from build123d import *

# Parameters (mm, degrees)
EXTRUDE_1_DEPTH     = 15
REVOLVE_1_ANGLE     = 180.0000000000004
CUT_EXTRUDE_START   = -19
CUT_EXTRUDE_1_DEPTH = 19
SKETCH_5_R          = 10
CUT_EXTRUDE_2_DEPTH = 87.34958022017247
SKETCH_4_R          = 1.2499999999999991
SKETCH_4_R_2        = 1.2500000000000002
SKETCH_4_R_3        = 1.2499999999999996
SKETCH_4_R_4        = 1.2499999999999987
SKETCH_4_R_5        = 1.2499999999999984
SKETCH_4_R_6        = 1.249999999999999
SKETCH_4_R_7        = 5.1000000000000005
CUT_EXTRUDE_3_DEPTH = 86.88509768172823
CUT_EXTRUDE_START_2 = -3
CUT_EXTRUDE_5_DEPTH = 3
SKETCH_6_R          = 6.200000000000004
CUT_EXTRUDE_4_DEPTH = 4.2
EXTRUDE_2_DEPTH     = 15
CHAMFER_1_SIZE      = 0.3
HOLE_WIZARD_1_D     = 1.7
HOLE_WIZARD_1_DEPTH = 3.5


with BuildPart() as part:
    # 草图2 → 凸台-拉伸1 (new body)
    with BuildSketch(Plane(origin=(0, 0, 0), x_dir=(1, 0, 0), z_dir=(0, 1, 0))):
        with BuildLine():
            Line((70.44642857142858, 12.492025517529665), (0.5357142857142793, 14.990430621035568))
            ThreePointArc((0.5357142857142791, 14.990430621035566), (-10.41547612244118, 10.79434375693384), (-14.99999999999997, 1.22e-15))
            Line((-15, 0), (82.5, -8.67e-15))
            ThreePointArc((82.5, -8.44e-15), (78.99528646411157, 8.679563435367664), (70.44642857142858, 12.492025517529667))
        make_face()
        with BuildLine():
            Line((82.5, -8.67e-15), (-15, 0))
            ThreePointArc((-14.999999999999998, 0), (-10.415476122441204, -10.794343756933866), (0.535714285714286, -14.990430621035598))
            Line((0.5357142857142848, -14.990430621035598), (70.44642857142858, -12.492025517529669))
            ThreePointArc((70.44642857142858, -12.492025517529669), (78.99528646411156, -8.679563435367672), (82.5, -8.72e-15))
        make_face()
    extrude(amount=EXTRUDE_1_DEPTH)

    # 草图1 → 旋转1 (revolve)
    with BuildSketch(Plane(origin=(0, 0, 0), x_dir=(1, 0, 0), z_dir=(0, 1, 0))):
        with BuildLine():
            Line((0.5357142857142848, -14.990430621035598), (70.44642857142858, -12.492025517529669))
            ThreePointArc((70.44642857142858, -12.492025517529669), (78.99528646411156, -8.67956343536767), (82.5, 0))
            Line((82.5, 0), (-15, 0))
            ThreePointArc((-15, 0), (-10.415476122441207, -10.794343756933864), (0.5357142857142848, -14.990430621035598))
        make_face()
    revolve(axis=Axis((70, 0, 8.67e-15), (1, 0, 1.2e-16)), revolution_arc=REVOLVE_1_ANGLE)

    # 草图3 → 切除-拉伸1 (cut)
    with BuildSketch(Plane(origin=(0, 15, 0), x_dir=(1, 0, 0), z_dir=(0, 1, 0)).offset(CUT_EXTRUDE_START)):
        with BuildLine():
            Line((17.295525226029294, 14.391483841348133), (0.5357142857142793, 14.990430621035568))
            ThreePointArc((0.5357142857142793, 14.990430621035568), (-14.999999999999972, 1.84e-15), (0.5357142857142814, -14.990430621035584))
            Line((0.5357142857142814, -14.990430621035584), (17.29552522602928, -14.391483841348148))
            ThreePointArc((17.29552522602928, -14.391483841348148), (22.5, -9.99e-15), (17.295525226029294, 14.391483841348133))
        make_face()
    extrude(amount=CUT_EXTRUDE_1_DEPTH, mode=Mode.SUBTRACT)

    # 草图5 → 切除-拉伸2 (cut, through all)
    with BuildSketch(Plane(origin=(0, -6, 0), x_dir=(1, 0, 0), z_dir=(0, 1, 0))):
        with Locations(Location((0, 0, 0), (0, 0, 270))):
            Circle(SKETCH_5_R)
    extrude(amount=-CUT_EXTRUDE_2_DEPTH, mode=Mode.SUBTRACT)

    # 草图4 → 切除-拉伸3 (cut, through all)
    with BuildSketch(Plane(origin=(0, -4, 0), x_dir=(1, 0, 0), z_dir=(0, 1, 0))):
        with Locations(Location((8, 0, 0), (0, 0, 270))):
            Circle(SKETCH_4_R)
        with Locations(Location((5.656854249492371, -5.656854249492391, 0), (0, 0, 270))):
            Circle(SKETCH_4_R_2)
        with Locations(Location((-2.793e-14, -8, 0), (0, 0, 270))):
            Circle(SKETCH_4_R_3)
        with Locations(Location((-5.656854249492411, -5.65685424949235, 0), (0, 0, 270))):
            Circle(SKETCH_4_R_4)
        with Locations(Location((-8, 5.586e-14, 0), (0, 0, 270))):
            Circle(SKETCH_4_R_5)
        with Locations(Location((-5.65685424949233, 5.656854249492429, 0), (0, 0, 270))):
            Circle(SKETCH_4_R_3)
        with Locations(Location((8.38e-14, 7.999999999999998, 0), (0, 0, 270))):
            Circle(SKETCH_4_R_6)
        with Locations(Location((5.656854249492451, 5.656854249492311, 0), (0, 0, 270))):
            Circle(SKETCH_4_R_6)
        with Locations(Location((0, 0, 0), (0, 0, 270))):
            Circle(SKETCH_4_R_7)
    extrude(amount=-CUT_EXTRUDE_3_DEPTH, mode=Mode.SUBTRACT)

    # 草图11 → 切除-拉伸5 (cut)
    with BuildSketch(Plane(origin=(0, 15, 0), x_dir=(1, 0, 0), z_dir=(0, 1, 0)).offset(CUT_EXTRUDE_START_2)):
        with BuildLine():
            Line((60.46530800021301, 12.848721666733917), (70.44642857142858, 12.492025517529665))
            ThreePointArc((70.44642857142858, 12.492025517529665), (82.5, -8.67e-15), (70.44642857142858, -12.492025517529669))
            Line((70.44642857142858, -12.492025517529669), (60.46530800021299, -12.848721666733926))
            ThreePointArc((60.46530800021299, -12.848721666733926), (54, 3.9e-16), (60.46530800021301, 12.848721666733917))
        make_face()
    extrude(amount=CUT_EXTRUDE_5_DEPTH, mode=Mode.SUBTRACT)

    # 草图6 → 切除-拉伸4 (cut)
    with BuildSketch(Plane(origin=(0, 12, 0), x_dir=(1, 0, 0), z_dir=(0, 1, 0))):
        with Locations(Location((70, -8.67e-15, 0), (0, 0, 270))):
            Circle(SKETCH_6_R)
    extrude(amount=-CUT_EXTRUDE_4_DEPTH, mode=Mode.SUBTRACT)

    # 草图12 → 凸台-拉伸2 (add)
    with BuildSketch(Plane(origin=(0, 15, 0), x_dir=(1, 0, 0), z_dir=(0, 1, 0))):
        Polygon((38.755416613121156, 10.122335609132724), (38.59470232740688, 5.625206422822045), (46.58959865862586, 5.339492137107765), (46.750312944340145, 9.836621323418441), align=None)
        Polygon((30.760520281902174, 10.408049894847004), (30.59980599618789, 5.910920708536326), (38.59470232740688, 5.625206422822045), (38.755416613121156, 10.122335609132724), align=None)
    extrude(amount=EXTRUDE_2_DEPTH)

    # 倒角1
    chamfer_1_edges = [part.edges().sort_by_distance(p)[0] for p in [
        (38.755416613121156, 30, -10.122335609132723),
        (30.680163139045032, 30, -8.159485301691664),
        (38.59470232740688, 30, -5.625206422822045),
        (46.669955801483, 30, -7.588056730263103),
    ]]
    chamfer(chamfer_1_edges, length=CHAMFER_1_SIZE)

    # 孔1
    with Locations(Plane(origin=(0.41071428571427876, 0, -11.492663476127266), x_dir=(-0.9993620414023731, 0, -0.03571428571428518), z_dir=(0.03571428571428518, 0, -0.9993620414023731))):
        with Locations((-41.369180272, 27.499999998), (-35.369180272, 27.499999998)):
            Hole(HOLE_WIZARD_1_D / 2, depth=HOLE_WIZARD_1_DEPTH)


solid = part.part
Geometry check sheet. Reference: the model listing, model coordinates, mm. A direction names the side the tool comes from. Give positions to 0.01 mm unless a question says otherwise; leave off trailing zeros. Write each loop counter-clockwise with the first axis right and the second up, starting at its lowest first coordinate (ties: lowest second). Pieces come first, ordered by that corner, then holes.
1) Cross-section at A-A (z = 0). Record the boundary of the cut face in (x, y).
Values follow:
outline: (-14.46, -4) arc R15 ccw to (-10, -11.18) - (-10, -6) - (-9.25, -6) - (-9.25, -4) - close; (-6.75, -6) - (-5.1, -6) - (-5.1, -4) - (-6.75, -4) - close; (5.1, -6) - (6.75, -6) - (6.75, -4) - (5.1, -4) - close; (9.25, -6) - (10, -6) - (10, -14.65) - (70.45, -12.49) arc R12.5 ccw to (82.5, 0) - (82.5, 12) - (76.2, 12) - (76.2, 7.8) - (63.8, 7.8) - (63.8, 12) - (54, 12) - (54, 15) - (22.5, 15) - (22.5, -4) - (9.25, -4) - close
2) Thickness scan on line 1 (X direction, y = 10, z = 3.5); line 2 (X direction, y = 10, z = 0); line 3 (Y direction, x = 13.5, z = -2). Record the ranges inside material, lowest first.
Values follow:
line 1: x = 22.23 to 64.88, 75.12 to 82
line 2: x = 22.5 to 63.8, 76.2 to 82.5
line 3: y = -14.39 to -4
3) Release check for a two-part mould opening along Y. For faces 1 (the face through (4.437, -4.986, 5.386)), 2 (the face through (2, -6, -5)), 3 (the face through (42.082, 26.746, -8.228)) record: released by +Y, released by -Y, zero draft, split by the parting line, or undercut.
Values follow:
face 1: zero draft
face 2: released by -Y
face 3: undercut
4) Cross-section at D-D (z = -8). Count the separate pieces of the cut face and the enclosed holes in it, plus the area to 3 significant figures.
Values follow:
separate pieces: 2
enclosed holes: 2
area: 1,810 mm2
5) Cross-section at B-B (x = 21). Record the boundary of the cut face in (y, z).
Values follow:
outline: (-4, -8.08) - (-4, 8.08) - (15, 8.08) - (15, 14.26) - (0, 14.26) arc R14.26 ccw to (0, -14.26) - (15, -14.26) - (15, -8.08) - close
6) Go/stop test with flat-tipped pins: pin 1 Ø11.5 at (x, z) = (0, 0) entering from +Y; pin 2 Ø4 at (x, z) = (19, 10.5) entering from +Y; pin 3 Ø13 at (x, z) = (66, 5.5) entering from +Y. Record where each tip stops, or that it passes through.
Values follow:
pin 1: stops at y = -4
pin 2: stops at y = 15
pin 3: stops at y = 12
7) Cross-section at C-C (y = 22). Record the boundary of the cut face in (x, z).
Values follow:
outline: (30.6, -5.91) - (30.76, -10.41) - (46.75, -9.84) - (46.59, -5.34) - close
8) Set-up check for faces 4 (the face through (82.497, 5.916, 0.269)), 5 (the face through (62, 12, 0)), 6 (the face through (-4.603, -4.986, 6.329)), 7 (the face through (76.147, 9.929, -0.807)), 8 (the face through (22.5, 5.4, 0.2)): record each of +Z, -Z, +X, -X, +Y, -Y from which the full face is reachable in a straight line by a thin tool's end or side.
Values follow:
face 4: +X, +Y, -Y
face 5: +X, +Y
face 6: +Y, -Y
face 7: +Y
face 8: -X, +Y
